Here's the drawing with two shaded views (mm, measured from the low corner). I have some questions. A direction names the side the tool comes from. Give positions to 0.01 mm unless a question says otherwise; leave off trailing zeros. Loops run counter-clockwise (first coordinate to the right, second up) from the corner with the lowest first, then second, coordinate; pieces in that order, holes last. Notation, with made-up numbers: M 79.5,24 L 91.5,24 A26 ccw 91.5,62 Z; hole C 32.5,74.25 d4. An arc over 180 degrees is marked long. Use CSV: the item, a comma, the result in double quotes.
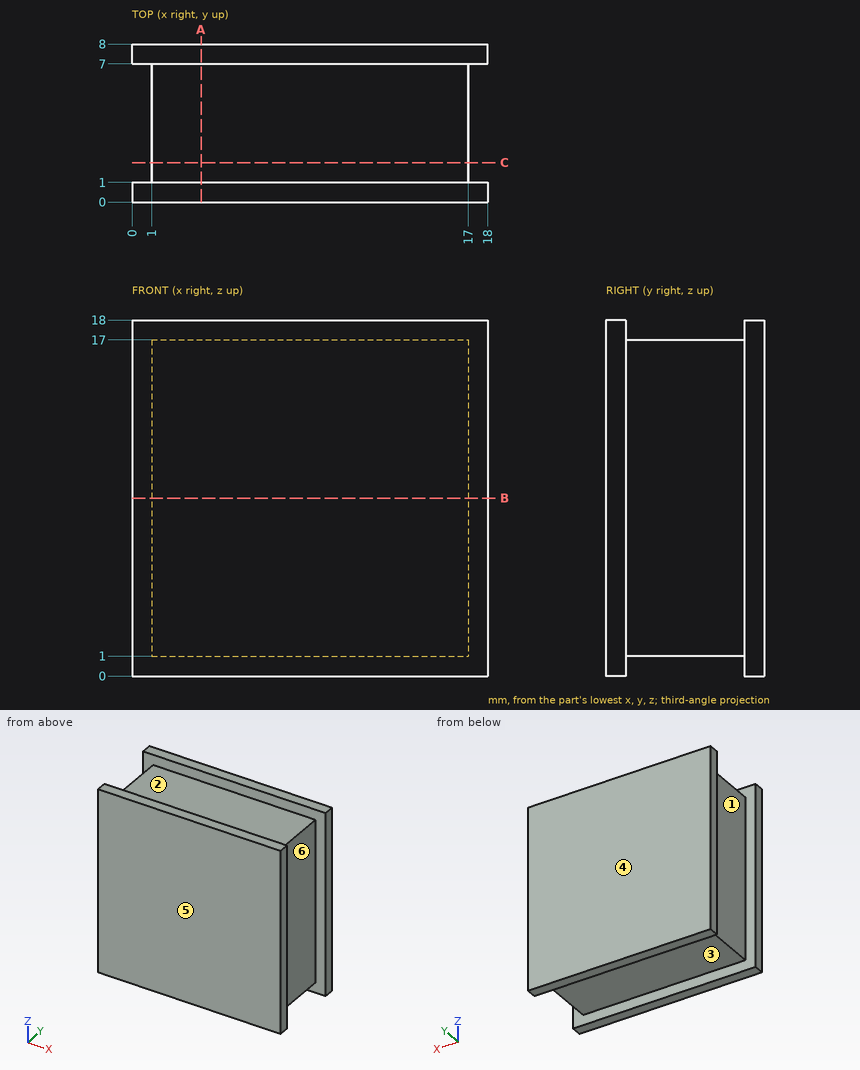
1. I want a section at C-C, the plane y = 2. List the corners of the cut face in (x, z) for me, then the cut area to 3 significant figures.
Outcome:
outline,"M 1,1 L 17,1 L 17,17 L 1,17 Z"
area,"256 mm2"
2. I want a section at B-B, the plane z = 9. List the corners of the cut face in (x, y) for me, then the cut area to 3 significant figures.
Outcome:
outline,"M 0,0 L 18,0 L 18,1 L 17,1 L 17,7 L 18,7 L 18,8 L 0,8 L 0,7 L 1,7 L 1,1 L 0,1 Z"
area,"132 mm2"
3. Please list where these lines run through material, in increasing order: line 1 (Y direction, x = 17.25, z = 8); line 2 (Z direction, x = 11, y = 6).
Outcome:
line 1,"0 to 1, 7 to 8"
line 2,"1 to 17"
4. I want a section at A-A, the plane x = 3.5. List the corners of the cut face in (y, z) for me, then the cut area to 3 significant figures.
Outcome:
outline,"M 0,0 L 1,0 L 1,1 L 7,1 L 7,0 L 8,0 L 8,18 L 7,18 L 7,17 L 1,17 L 1,18 L 0,18 Z"
area,"132 mm2"
5. If we mould it in two halves opening along Y, with no side actions, what happens to the marked faces 4, 5 and 6? For each: +Y half, -Y half, draft (parallel to the pull), parting line (faces both ways), or undercut.
Outcome:
face 4,"+Y half"
face 5,"-Y half"
face 6,"undercut"
6. I'm going to push a flat-ended pin straight in: pin 1 Ø1 at (x, y) = (9, 2) entering from +Z. Where does the tip first touch, or does it pass through?
Outcome:
pin 1,"z = 17"
7. Which directions (+Z, -Z, +X, -X, +Y, -Y) give clear straight access to the entire face, cutting with the end or side of a thin tool? Please do the marked faces 1, 2 and 3.
Outcome:
face 1,"+Z, -Z, -X"
face 2,"+Z, +X, -X"
face 3,"-Z, +X, -X"
